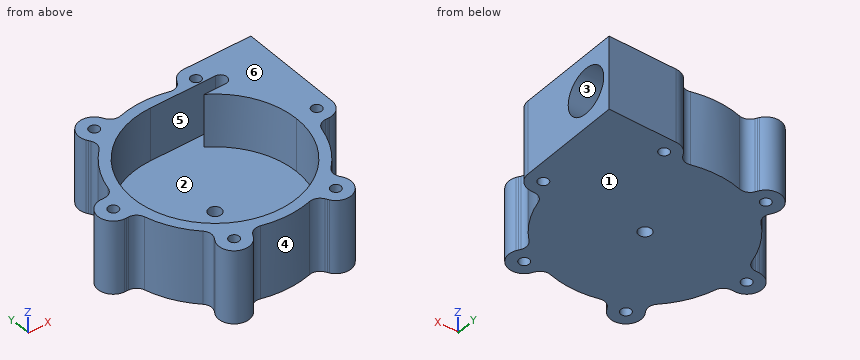
```python
from build123d import *

# Parameters (mm, degrees)
F0_R     = 1.25
F1_DEPTH = 18
F3_D     = 11.13
F3_DEPTH = 12.5
F3_TIP   = 3.3437893449
F4_R     = 1.5625
F5_DEPTH = 5


with BuildPart() as f1:
    # F0 (on Top) → F1 (new body)
    with BuildSketch(Plane.XY):
        with BuildLine():
            ThreePointArc((-15.3434944638, 19.0939042011), (-15.0320560296, 17.5061736151), (-15.7581247751, 16.060246062))
            ThreePointArc((-15.7581247751, 16.060246062), (-19.4845549428, 11.2517606925), (-21.7866280292, 5.620750761))
            ThreePointArc((-21.7866280292, 5.620750761), (-22.6760479277, 4.2691537219), (-24.2068768675, 3.7452786709))
            Line((-24.2068768675, 3.7452786709), (-24.8095572627, 3.7451611218))
            Line((-24.8095572627, 3.7451611218), (-25.1919036634, 3.7450865475))
            ThreePointArc((-25.1919036634, 3.7450865475), (-28.7498129399, 0.0374555534), (-25.2666745248, -3.7405059061))
            Line((-25.2666745248, -3.7405059061), (-24.7361366604, -3.7407052642))
            Line((-24.7361366604, -3.7407052642), (-24.2075533275, -3.7409038879))
            ThreePointArc((-24.2075533275, -3.7409038879), (-22.6768190885, -4.2650555852), (-21.7876434683, -5.6168133403))
            ThreePointArc((-21.7876434683, -5.6168133403), (-19.4865880684, -11.2482392157), (-15.761026962, -16.0573979556))
            ThreePointArc((-15.761026962, -16.0573979556), (-15.0352195396, -17.5034567019), (-15.346944907, -19.0911309781))
            Line((-15.346944907, -19.0911309781), (-15.6481833041, -19.6131262852))
            Line((-15.6481833041, -19.6131262852), (-15.8392919213, -19.9442852685))
            ThreePointArc((-15.8392919213, -19.9442852685), (-14.4073439307, -24.8793405833), (-9.3939641247, -23.7518349607))
            Line((-9.3939641247, -23.7518349607), (-9.1285225433, -23.2924753715))
            Line((-9.1285225433, -23.2924753715), (-8.8640588637, -22.834808089))
            ThreePointArc((-8.8640588637, -22.834808089), (-7.6447630589, -21.7712292003), (-6.0295186932, -21.6770594023))
            ThreePointArc((-6.0295186932, -21.6770594023), (-0.0020331256, -22.4999999081), (6.0256010672, -21.6781487166))
            ThreePointArc((6.0256010672, -21.6781487166), (7.640828388, -21.7726104237), (8.8599319605, -22.836409649))
            Line((8.8599319605, -22.836409649), (9.1613739586, -23.358287407))
            Line((9.1613739586, -23.358287407), (9.3526117422, -23.689371816))
            ThreePointArc((9.3526117422, -23.689371816), (14.3424690092, -24.9167961367), (15.8727104001, -20.0113290546))
            Line((15.8727104001, -20.0113290546), (15.6076141171, -19.5517701073))
            Line((15.6076141171, -19.5517701073), (15.3434944638, -19.0939042011))
            ThreePointArc((15.3434944638, -19.0939042011), (15.0320560296, -17.5061736151), (15.7581247751, -16.060246062))
            ThreePointArc((15.7581247751, -16.060246062), (19.4845549428, -11.2517606925), (21.7866280292, -5.620750761))
            ThreePointArc((21.7866280292, -5.620750761), (22.6760479277, -4.2691537219), (24.2068768675, -3.7452786709))
            Line((24.2068768675, -3.7452786709), (24.8095572627, -3.7451611218))
            Line((24.8095572627, -3.7451611218), (25.1919036634, -3.7450865475))
            ThreePointArc((25.1919036634, -3.7450865475), (27.7059534295, -2.5962118983), (28.7498196477, -0.0367778781))
            Line((28.7498196477, -0.0367778781), (28.9992988817, 25.3997910768))
            Line((28.9992988817, 25.3997910768), (12.5795568592, 25.3997910768))
            ThreePointArc((12.5795568592, 25.3997910768), (10.7769696358, 24.9813506545), (9.3939641247, 23.7518349607))
            Line((9.3939641247, 23.7518349607), (9.1285225433, 23.2924753715))
            Line((9.1285225433, 23.2924753715), (8.8640588637, 22.834808089))
            ThreePointArc((8.8640588637, 22.834808089), (7.6447630589, 21.7712292003), (6.0295186932, 21.6770594023))
            ThreePointArc((6.0295186932, 21.6770594023), (0.0020331256, 22.4999999081), (-6.0256010672, 21.6781487166))
            ThreePointArc((-6.0256010672, 21.6781487166), (-7.640828388, 21.7726104237), (-8.8599319605, 22.836409649))
            Line((-8.8599319605, 22.836409649), (-9.1613739586, 23.358287407))
            Line((-9.1613739586, 23.358287407), (-9.3526117422, 23.689371816))
            ThreePointArc((-9.3526117422, 23.689371816), (-14.3424690092, 24.9167961367), (-15.8727104001, 20.0113290546))
            Line((-15.8727104001, 20.0113290546), (-15.6076141171, 19.5517701073))
            Line((-15.6076141171, 19.5517701073), (-15.3434944638, 19.0939042011))
        make_face()
        with Locations((-12.5, -21.650635024)):
            Circle(F0_R, mode=Mode.SUBTRACT)
        with Locations((12.4999999694, -21.6506350416)):
            Circle(F0_R, mode=Mode.SUBTRACT)
        with Locations((-24.9999999694, 5.3e-08)):
            Circle(F0_R, mode=Mode.SUBTRACT)
        with BuildLine():
            ThreePointArc((10.7347275233, 16.875), (17.5313226892, 9.6256285388), (20, 0))
            ThreePointArc((20, 0), (-14.1421356237, -14.1421356237), (0, 20))
            Line((0, 20), (13.682886083, 20))
            Line((13.682886083, 20), (16, 20))
            ThreePointArc((16, 20), (17.5625, 18.4375), (16, 16.875))
            Line((16, 16.875), (13.7064243678, 16.875))
            Line((13.7064243678, 16.875), (10.7347275233, 16.875))
        make_face(mode=Mode.SUBTRACT)
        with Locations((-12.4999999694, 21.6506351123)):
            Circle(F0_R, mode=Mode.SUBTRACT)
        with Locations((24.9999999694, 1.77e-08)):
            Circle(F0_R, mode=Mode.SUBTRACT)
        with Locations((12.5, 21.6506350946)):
            Circle(F0_R, mode=Mode.SUBTRACT)
    extrude(amount=F1_DEPTH)

    # F3
    with Locations(Plane(origin=(28.7474150086, -0.2819516693, 0), x_dir=(0.0098074247, 0.9999519061, 0), z_dir=(0.9999519061, -0.0098074247, 0))):
        with Locations((18.4329779418, 9)):
            Hole(F3_D / 2, depth=F3_DEPTH)
            with Locations((0, 0, -(F3_DEPTH + F3_TIP / 2))):  # 118° drill point
                Cone(0, F3_D / 2, F3_TIP, mode=Mode.SUBTRACT)

    # F4 (on face) → F5 (join)
    with BuildSketch(Plane(origin=(0, 0, 0), x_dir=(1, 0, 0), z_dir=(0, 0, -1))):
        with BuildLine():
            ThreePointArc((10.7347275233, -16.875), (-5.5901699437, 19.2028643697), (0, -20))
            Line((0, -20), (16, -20))
            ThreePointArc((16, -20), (17.5625, -18.4375), (16, -16.875))
            Line((16, -16.875), (10.7347275233, -16.875))
        make_face()
        Circle(F4_R, mode=Mode.SUBTRACT)
    extrude(amount=-F5_DEPTH)


solid = f1.part
```
Input: part model. Units: mm. Frame: model coordinates. Face numbers are marked on the shaded views. A direction names the side the tool comes from. Round coordinates to 2 decimals unless told otherwise and drop trailing zeros. Order: outer loops, then holes, each group sorted by start corner. A loop starts at its lowest first (then second) coordinate and runs counter-clockwise, first axis right, second up. Notation, with made-up numbers: (14, -36.5) - (30, -36.5) arc R20 ccw to (30, -1.5) - close; hole circle Ø8 at (-9, -37). An arc over 180 degrees is marked (long way). One line per question, with ' | ' between items. Start each with the question number.
1) Cut plane C-C, the plane x = -18.5. Return the cut outline in (y, z).
2) Cut plane B-B, the plane y = -13. Return the cut outline in (x, z), then the cut area to 3 significant figures.
3) Ray query, probe 1 along Y at (x, z) = (-12.5, 8.25); probe 2 along Y at (x, z) = (0, 1.85); probe 3 along X at (y, z) = (-1, 5.75). Return the intervals inside material, ascending.
4) Cut plane A-A, the plane x = -12.5. Return the cut outline in (y, z).
5) Contact query for flat-ended pins moving along their axis: P1, Ø8, axis at y = 6.5, z = 3, coming from the +X side; P2, Ø10.5, axis at x = 9.5, z = 8.5, coming from the -Y side; P3, Ø2, axis at x = -7, z = 9.5, coming from the -Y side; P4, Ø2, axis at x = -6, y = -10, coming from the +Z side. Output: stop coordinate, or through.
6) Pull-direction query (Y, two-part tool) for the marked faces 1, 2, 3 and 4; classes: +Y half, -Y half, draft (parallel to the pull), parting line (faces both ways), or undercut.
7) Cut plane D-D, the plane z = 1.75. Give the number of separate pieces and of enclosed holes in the cut face, then the cut area to 3 significant figures.
8) Set-up query: the marked faces 5 and 6. Return all of +Z, -Z, +X, -X, +Y, -Y with unobstructed straight access to the full face (end or side cutting, diameter ignored); none if empty.
Worked out:
1) outline: (-12.81, 0) - (12.81, 0) - (12.81, 18) - (7.6, 18) - (7.6, 5) - (-7.6, 5) - (-7.6, 18) - (-12.81, 18) - close
2) outline: (-18.36, 0) - (18.36, 0) - (18.36, 18) - (15.2, 18) - (15.2, 5) - (-15.2, 5) - (-15.2, 18) - (-18.36, 18) - close | area: 266 mm^2
3) probe 1: y = -25.4 to -22.9, -20.4 to -15.61, 15.61 to 20.4, 22.9 to 25.4 | probe 2: y = -22.5 to -1.56, 1.56 to 22.5 | probe 3: x = -28.61 to -25.75, -24.25 to -19.97, 19.97 to 24.25, 25.75 to 28.61
4) outline: (-25.4, 0) - (-22.9, 0) - (-22.9, 18) - (-25.4, 18) - close; (-20.4, 0) - (20.4, 0) - (20.4, 18) - (15.61, 18) - (15.61, 5) - (-15.61, 5) - (-15.61, 18) - (-20.4, 18) - close; (22.9, 0) - (25.4, 0) - (25.4, 18) - (22.9, 18) - close
5) P1: stops at x = 28.85 | P2: stops at y = -25.4 | P3: stops at y = -21.95 | P4: stops at z = 5
6) face 1: draft | face 2: undercut | face 3: undercut | face 4: -Y half
7) separate pieces: 1 | enclosed holes: 7 | area: 2,050 mm^2
8) face 5: +Z | face 6: +Z, +X, -X, +Y, -Y
